from build123d import *

# Parameters (mm, degrees)
SKETCH1_W                = 118
SKETCH1_H                = 40
SKETCH1_W_2              = 11
BOSS_EXTRUDE1_DEPTH      = 3
BOSS_EXTRUDE2_START      = -5
SKETCH1_3_W              = 118
SKETCH1_3_H              = 40
BOSS_EXTRUDE2_DEPTH      = 5
FILLET1_R                = 5
BOSS_EXTRUDE3_DEPTH      = 4
LPATTERN1_COUNT          = 2
LPATTERN1_PITCH          = 22.5
LPATTERN1_COL_COUNT      = 2
LPATTERN1_COL_PITCH      = 22.5
M3_CLEARANCE_HOLE1_D     = 3.6
M3_CLEARANCE_HOLE1_DEPTH = 9
M3_CLEARANCE_HOLE1_TIP   = 1.081549114
CUT_EXTRUDE2_DEPTH       = 79.364532794
SKETCH12_W               = 5
SKETCH12_H               = 39.2
CUT_EXTRUDE3_DEPTH       = 0.3
SKETCH13_W               = 5
SKETCH13_H               = 39.2
CUT_EXTRUDE4_DEPTH       = 0.3
CUT_EXTRUDE5_START       = -0.3
CUT_EXTRUDE5_DEPTH       = 0.3
SKETCH16_W               = 14.5
SKETCH16_H               = 6.6
CUT_EXTRUDE7_DEPTH       = 3


# Read off the part's stored shape, not the designer's step: CSK for M3 Flat Head Machine Screw1
with BuildPart() as part:
    # Sketch1 → Boss-Extrude1 (new body)
    # profile 1 of 3: a face of its own
    with BuildSketch(Plane.XY):
        Rectangle(SKETCH1_W, SKETCH1_H)
        with BuildLine():
            ThreePointArc((-32.5, -13), (-45.5, 0), (-32.5, 13))
            Line((-32.5, 13), (32.5, 13))
            ThreePointArc((32.5, 13), (45.5, 0), (32.5, -13))
            Line((32.5, -13), (-32.5, -13))
        make_face(mode=Mode.SUBTRACT)
    # profile 2 of 3: a face of its own
    with BuildSketch(Plane.XY):
        with Locations((-64.5, 0)):
            Rectangle(SKETCH1_W_2, SKETCH1_H)
    # profile 3 of 3: a face of its own
    with BuildSketch(Plane.XY):
        with Locations((64.5, 0)):
            Rectangle(SKETCH1_W_2, SKETCH1_H)
    extrude(amount=BOSS_EXTRUDE1_DEPTH)

    # Sketch1<3> → Boss-Extrude2 (add)
    with BuildSketch(Plane.XY.offset(BOSS_EXTRUDE2_START)):
        Rectangle(SKETCH1_3_W, SKETCH1_3_H)
        with BuildLine():
            ThreePointArc((-32.5, -13), (-45.5, 0), (-32.5, 13))
            Line((-32.5, 13), (32.5, 13))
            ThreePointArc((32.5, 13), (45.5, 0), (32.5, -13))
            Line((32.5, -13), (-32.5, -13))
        make_face(mode=Mode.SUBTRACT)
    extrude(amount=BOSS_EXTRUDE2_DEPTH)

    # CSK for M3 Flat Head Machine Screw1 outl → CSK for M3 Flat Head Machine Screw1 (revolve, cut)
    with BuildSketch(Plane(origin=(65, 0, 0), x_dir=(1, 0, 0), z_dir=(0, -1, 0))):
        Polygon((0, 0), (1.8, 0), (1.8, 1.65), (3.15, 3), (0, 3), align=None)
    revolve(axis=Axis((65, 0, 0), (0, 0, 1)), mode=Mode.SUBTRACT)

    # CSK for M3 Flat Head Machine Screw1 2 ou → CSK for M3 Flat Head Machine Screw1 2 (revolve, cut)
    with BuildSketch(Plane(origin=(-65, 0, 0), x_dir=(1, 0, 0), z_dir=(0, -1, 0))):
        Polygon((0, 0), (1.8, 0), (1.8, 1.65), (3.15, 3), (0, 3), align=None)
    revolve(axis=Axis((-65, 0, 0), (0, 0, 1)), mode=Mode.SUBTRACT)

    # CSK for M3 Flat Head Machine Screw1 3 ou → CSK for M3 Flat Head Machine Screw1 3 (revolve, cut)
    with BuildSketch(Plane(origin=(-65, -15, 0), x_dir=(1, 0, 0), z_dir=(0, -1, 0))):
        Polygon((0, 0), (1.8, 0), (1.8, 1.65), (3.15, 3), (0, 3), align=None)
    revolve(axis=Axis((-65, -15, 0), (0, 0, 1)), mode=Mode.SUBTRACT)

    # CSK for M3 Flat Head Machine Screw1 4 ou → CSK for M3 Flat Head Machine Screw1 4 (revolve, cut)
    with BuildSketch(Plane(origin=(65, 15, 0), x_dir=(1, 0, 0), z_dir=(0, -1, 0))):
        Polygon((0, 0), (1.8, 0), (1.8, 1.65), (3.15, 3), (0, 3), align=None)
    revolve(axis=Axis((65, 15, 0), (0, 0, 1)), mode=Mode.SUBTRACT)

    # CSK for M3 Flat Head Machine Screw1 5 ou → CSK for M3 Flat Head Machine Screw1 5 (revolve, cut)
    with BuildSketch(Plane(origin=(65, -15, 0), x_dir=(1, 0, 0), z_dir=(0, -1, 0))):
        Polygon((0, 0), (1.8, 0), (1.8, 1.65), (3.15, 3), (0, 3), align=None)
    revolve(axis=Axis((65, -15, 0), (0, 0, 1)), mode=Mode.SUBTRACT)

    # CSK for M3 Flat Head Machine Screw1 6 ou → CSK for M3 Flat Head Machine Screw1 6 (revolve, cut)
    with BuildSketch(Plane(origin=(-65, 15, 0), x_dir=(1, 0, 0), z_dir=(0, -1, 0))):
        Polygon((0, 0), (1.8, 0), (1.8, 1.65), (3.15, 3), (0, 3), align=None)
    revolve(axis=Axis((-65, 15, 0), (0, 0, 1)), mode=Mode.SUBTRACT)

    # Fillet1
    fillet1_edges = [part.edges().sort_by_distance(p)[0] for p in [
        (-70, -20, 1.5),
        (-70, 20, 1.5),
        (70, 20, 1.5),
        (70, -20, 1.5),
    ]]
    fillet(fillet1_edges, radius=FILLET1_R)

    # Sketch5 → Boss-Extrude3 (add, symmetric)
    with BuildSketch(Plane(origin=(0, 0, 0), x_dir=(0, 0, -1), z_dir=(1, 0, 0))):
        Polygon((5, -13), (5, -20), (26, -20), (26, 20), (5, 20), (5, 13), (22, 13), (22, -13), align=None)
    boss_extrude3 = extrude(amount=BOSS_EXTRUDE3_DEPTH, both=True)

    # LPattern1: Boss-Extrude3 ×2
    with Locations(*[(i * LPATTERN1_PITCH, 0, 0) for i in range(1, LPATTERN1_COUNT)]):
        add(boss_extrude3)

    # LPattern1 col: Boss-Extrude3 ×2
    with Locations(*[(-i * LPATTERN1_COL_PITCH, 0, 0) for i in range(1, LPATTERN1_COL_COUNT)]):
        add(boss_extrude3)

    # M3 Clearance Hole1
    with Locations(Plane(origin=(0, 0, -26), x_dir=(-1, 0, 0), z_dir=(0, 0, -1))):
        with Locations((-22.5, 0), (22.5, 0)):
            Hole(M3_CLEARANCE_HOLE1_D / 2, depth=M3_CLEARANCE_HOLE1_DEPTH)
            with Locations((0, 0, -(M3_CLEARANCE_HOLE1_DEPTH + M3_CLEARANCE_HOLE1_TIP / 2))):  # 118° drill point
                Cone(0, M3_CLEARANCE_HOLE1_D / 2, M3_CLEARANCE_HOLE1_TIP, mode=Mode.SUBTRACT)

    # Sketch10 → Cut-Extrude2 (cut, through all)
    with BuildSketch(Plane.XY.offset(3)):
        with BuildLine():
            Line((70, -15), (70, 15))
            ThreePointArc((70, 15), (68.535533906, 18.535533906), (65, 20))
            Line((65, 20), (-65, 20))
            ThreePointArc((-65, 20), (-68.535533906, 18.535533906), (-70, 15))
            Line((-70, 15), (-70, -15))
            ThreePointArc((-70, -15), (-68.535533906, -18.535533906), (-65, -20))
            Line((-65, -20), (65, -20))
            ThreePointArc((65, -20), (68.535533906, -18.535533906), (70, -15))
        make_face()
        with BuildLine():
            Line((69.6, -15), (69.6, 15))
            ThreePointArc((69.6, 15), (68.252691193, 18.252691193), (65, 19.6))
            Line((65, 19.6), (-65, 19.6))
            ThreePointArc((-65, 19.6), (-68.252691193, 18.252691193), (-69.6, 15))
            Line((-69.6, 15), (-69.6, -15))
            ThreePointArc((-69.6, -15), (-68.252691193, -18.252691193), (-65, -19.6))
            Line((-65, -19.6), (65, -19.6))
            ThreePointArc((65, -19.6), (68.252691193, -18.252691193), (69.6, -15))
        make_face(mode=Mode.SUBTRACT)
    extrude(amount=-CUT_EXTRUDE2_DEPTH, mode=Mode.SUBTRACT)

    # Sketch12 → Cut-Extrude3 (cut)
    with BuildSketch(Plane(origin=(59, 0, 0), x_dir=(0, 0, -1), z_dir=(1, 0, 0))):
        with Locations((2.5, 0)):
            Rectangle(SKETCH12_W, SKETCH12_H)
    extrude(amount=-CUT_EXTRUDE3_DEPTH, mode=Mode.SUBTRACT)

    # Sketch13 → Cut-Extrude4 (cut)
    with BuildSketch(Plane.ZY.offset(59)):
        with Locations((-2.5, 0)):
            Rectangle(SKETCH13_W, SKETCH13_H)
    extrude(amount=-CUT_EXTRUDE4_DEPTH, mode=Mode.SUBTRACT)

    # Sketch14 → Cut-Extrude5 (cut)
    with BuildSketch(Plane(origin=(0, 0, 0), x_dir=(-1, 0, 0), z_dir=(0, 0, -1)).offset(CUT_EXTRUDE5_START)):
        with BuildLine():
            Line((-65, -19.6), (-58.7, -19.6))
            Line((-58.7, -19.6), (-58.7, 19.6))
            Line((-58.7, 19.6), (-65, 19.6))
            ThreePointArc((-65, 19.6), (-68.252691193, 18.252691193), (-69.6, 15))
            Line((-69.6, 15), (-69.6, -15))
            ThreePointArc((-69.6, -15), (-68.252691193, -18.252691193), (-65, -19.6))
        make_face()
        with BuildLine():
            Line((58.7, -19.6), (65, -19.6))
            ThreePointArc((65, -19.6), (68.252691193, -18.252691193), (69.6, -15))
            Line((69.6, -15), (69.6, 15))
            ThreePointArc((69.6, 15), (68.252691193, 18.252691193), (65, 19.6))
            Line((65, 19.6), (58.7, 19.6))
            Line((58.7, 19.6), (58.7, -19.6))
        make_face()
    extrude(amount=CUT_EXTRUDE5_DEPTH, mode=Mode.SUBTRACT)

    # Sketch16 → Cut-Extrude7 (cut)
    with BuildSketch(Plane(origin=(0, 0, -5), x_dir=(-1, 0, 0), z_dir=(0, 0, -1))):
        with Locations((11.25, 16.3)):
            Rectangle(SKETCH16_W, SKETCH16_H)
        with BuildLine():
            Line((58.7, -19.6), (58.7, 19.6))
            Line((58.7, 19.6), (26.5, 19.6))
            Line((26.5, 19.6), (26.5, 13))
            Line((26.5, 13), (32.5, 13))
            ThreePointArc((32.5, 13), (45.5, 0), (32.5, -13))
            Line((32.5, -13), (26.5, -13))
            Line((26.5, -13), (26.5, -19.6))
            Line((26.5, -19.6), (58.7, -19.6))
        make_face()
        with Locations((11.25, -16.3)):
            Rectangle(SKETCH16_W, SKETCH16_H)
        with Locations((-11.25, -16.3)):
            Rectangle(SKETCH16_W, SKETCH16_H)
        with Locations((-11.25, 16.3)):
            Rectangle(SKETCH16_W, SKETCH16_H)
        with BuildLine():
            Line((-58.7, 19.6), (-58.7, -19.6))
            Line((-58.7, -19.6), (-26.5, -19.6))
            Line((-26.5, -19.6), (-26.5, -13))
            Line((-26.5, -13), (-32.5, -13))
            ThreePointArc((-32.5, -13), (-45.5, 0), (-32.5, 13))
            Line((-32.5, 13), (-26.5, 13))
            Line((-26.5, 13), (-26.5, 19.6))
            Line((-26.5, 19.6), (-58.7, 19.6))
        make_face()
    extrude(amount=-CUT_EXTRUDE7_DEPTH, mode=Mode.SUBTRACT)


solid = part.part
Could you check a few things on this model? Use its own coordinates, in mm. A direction names the side the tool comes from. Give positions to 0.01 mm unless a question says otherwise; leave off trailing zeros. Order: outer loops, then holes, each group sorted by start corner. A loop starts at its lowest first (then second) coordinate and runs counter-clockwise, first axis right, second up.
1. For faces 1 (the flat face through (0, 13, -7)), 2 (the flat face through (63, 0, 0.3)), 3 (the flat face through (-26.5, 4.6, -22.2)), which set-ups out of +Z, -Z, +X, -X, +Y, -Y let a thin tool reach every point of the face, with its end or its side?
2. I need wall thicknesses on L1, parallel to Y at x = 65, z = 1.35; L2, parallel to X at y = -15, z = -9; L3, parallel to Y at x = 22.5, z = -23.05. Which ranges of each line are inside material? Lowest first, please.
3. Suppose I cut it at A-A (x = 8). List the corners of the cut face in (y, z) for me.
4. We'd pull the mould along Y, two halves only. Please class faces 4 (the cylindrical face through (45.497, 0.286, 0.465)), 5 (the flat face through (26.5, 5, -24)), 6 (the flat face through (0, 19.6, -5)): pulls with the +Y half, pulls with the -Y half, needs draft (parallel to the pull), parting line crosses it, or undercut.
5. Suppose I cut it at C-C (x = 22.5). List the corners of the cut face in (y, z) for me.
6. Suppose I cut it at D-D (y = -9.5). List the corners of the cut face in (x, z) for me.
7. Suppose I cut it at B-B (z = -11.75). List the corners of the cut face in (x, y) for me.
8. Will these pins go through, and if not, where does the flat tip stop? P1, Ø12, axis at y = -3.5, z = -9.5, coming from the -X side; P2, Ø12, axis at y = -9, z = -8.5, coming from the -X side; P3, Ø2, axis at x = -55, y = 3, coming from the -Z side; P4, Ø2.5, axis at y = 1, z = -1, coming from the -X side.
Solved:
1. face 1: +Z
1. face 2: -Z, +X, +Y, -Y
1. face 3: -Z, -X, +Y, -Y
2. L1: y = -19.6 to -16.8, -13.2 to -1.8, 1.8 to 13.2, 16.8 to 19.6
2. L2: x = -26.5 to -18.5, -4 to 4, 18.5 to 26.5
2. L3: y = -19.6 to -1.8, 1.8 to 19.6
3. outline: (-19.6, -2) - (-13, -2) - (-13, 3) - (-19.6, 3) - close; (13, -2) - (19.6, -2) - (19.6, 3) - (13, 3) - close
4. face 4: undercut
4. face 5: needs draft
4. face 6: pulls with the +Y half
5. outline: (-19.6, -26) - (-1.8, -26) - (-1.8, -22) - (-13, -22) - (-13, 3) - (-19.6, 3) - close; (1.8, -26) - (19.6, -26) - (19.6, 3) - (13, 3) - (13, -22) - (1.8, -22) - close
6. outline: (-69.6, 0.3) - (-58.7, 0.3) - (-58.7, -2) - (-41.37, -2) - (-41.37, 3) - (-69.6, 3) - close; (-26.5, -26) - (-18.5, -26) - (-18.5, -22) - (-26.5, -22) - close; (-4, -26) - (4, -26) - (4, -22) - (-4, -22) - close; (18.5, -26) - (26.5, -26) - (26.5, -22) - (18.5, -22) - close; (41.37, -2) - (58.7, -2) - (58.7, 0.3) - (69.6, 0.3) - (69.6, 3) - (41.37, 3) - close
7. outline: (-26.5, -19.6) - (-18.5, -19.6) - (-18.5, -13) - (-26.5, -13) - close; (-26.5, 13) - (-18.5, 13) - (-18.5, 19.6) - (-26.5, 19.6) - close; (-4, -19.6) - (4, -19.6) - (4, -13) - (-4, -13) - close; (-4, 13) - (4, 13) - (4, 19.6) - (-4, 19.6) - close; (18.5, -19.6) - (26.5, -19.6) - (26.5, -13) - (18.5, -13) - close; (18.5, 13) - (26.5, 13) - (26.5, 19.6) - (18.5, 19.6) - close
8. P1: passes through
8. P2: stops at x = -26.5
8. P3: stops at z = -2
8. P4: stops at x = -58.7
